Autodesk Inventor part; units mm, degrees
ref_plane "YZ Plane" through (0, 0, 0) normal (1, 0, 0) x (0, 1, 0)
ref_plane "XZ Plane" through (0, 0, 0) normal (0, 1, 0) x (-1, 0, 0)
ref_plane "XY Plane" through (0, 0, 0) normal (0, 0, 1) x (1, 0, 0)
sketch "Sketch1" plane through (0, 0, 0) normal (0, 0, 1) x (1, 0, 0)
  line L0 (-20.935, 3.75) -> (20.935, 3.75)
  line L1 (20.935, 3.75) -> (20.935, -3.75)
  line L2 (20.935, -3.75) -> (-20.935, -3.75)
  line L3 (-20.935, -3.75) -> (-20.935, 3.75)
  line L4 (-20.935, 3.75) -> (20.935, -3.75) construction
  line L5 (20.935, 3.75) -> (-20.935, -3.75) construction
  point P0 (0, 0)
  dimension "d0" = 41.87
  dimension "d1" = 7.5
extrude "Extrusion1" add sketch "Sketch1" along normal mid plane 35.5
sketch "Sketch2" plane through (-20.935, -3.75, 17.75) normal (0, -1, 0) x (1, 0, 0)
  line L0 (0, -35.5) -> (0, 0)
  line L1 (0, -35.5) -> (0, -29.307)
  line L2 (0, -29.307) -> (5, -29.307)
  line L3 (5, -29.307) -> (5, -6.193)
  line L4 (5, -6.193) -> (41.87, -6.193)
  line L5 (41.87, -6.193) -> (41.87, -29.307)
  line L6 (41.87, -29.307) -> (5, -29.307)
  point P0 (20.935, -17.75)
  dimension "d4" = 6.193
  dimension "d5" = 5
  dimension "d6" = 23.114
  dimension "d7" = 36.87
extrude "Extrusion2" cut sketch "Sketch2" against normal blind 1.6
sketch "Sketch3" plane through (-20.935, -2.15, 17.75) normal (0, -1, 0) x (1, 0, 0)
  line L0 (5, -29.307) -> (5, -6.193)
  line L1 (5, -29.307) -> (5, -21.75)
  line L2 (5, -21.75) -> (5, -13.75)
  line L3 (5, -13.75) -> (40, -13.75)
  line L4 (40, -13.75) -> (40, -21.75)
  line L5 (40, -21.75) -> (5, -21.75)
  point P0 (20.935, -17.75)
  dimension "d10" = 7.557
  dimension "d11" = 8
  dimension "d12" = 35
extrude "Extrusion3" cut sketch "Sketch3" against normal blind 1.6
fillet "Fillet1" radius 5 2 edges at (0, 3.75, 17.75) (0, 3.75, -17.75)
fillet "Fillet2" radius 5 5 edges at (20.935, 2.2855, -16.2855) (20.935, -2.5, -17.75) (20.935, 2.2855, 16.2855) (20.935, -2.5, 17.75) (20.935, 3.75, 0)
sketch "Sketch5" plane through (-20.935, -0.55, 17.75) normal (0, -1, 0) x (1, 0, 0)
  line L0 (5, -29.307) -> (5, -21.75)
  line L1 (5, -21.75) -> (5, -20.85)
  line L2 (5, -29.307) -> (5, -6.193)
  line L3 (5, -20.85) -> (7.25, -20.85)
  line L4 (7.25, -20.85) -> (7.25, -14.65)
  line L5 (7.25, -14.65) -> (27.75, -14.65)
  line L6 (27.75, -14.65) -> (27.75, -20.85)
  line L7 (27.75, -20.85) -> (7.25, -20.85)
  point P0 (20.935, -17.75)
  dimension "d22" = 0.9
  dimension "d23" = 2.25
  dimension "d24" = 6.2
  dimension "d25" = 20.5
extrude "Extrusion5" cut sketch "Sketch5" against normal through all
sketch "Sketch6" plane through (-20.935, -3.75, -17.75) normal (0, -1, 0) x (1, 0, 0)
  line L0 (0, 0) -> (0, 35.5)
  line L1 (0, 35.5) -> (-15, 35.5)
  line L2 (-15, 35.5) -> (-15, 0)
  line L3 (-15, 0) -> (0, 0)
  line L4 (0, 0) -> (0, 35.5)
  point P0 (20.935, 17.75)
  dimension "d28" = 15
  dimension "d29" = 35.5
extrude "Extrusion6" add sketch "Sketch6" against normal blind 7.5
fillet "Fillet3" [suppressed]
sketch "Sketch7" plane through (0, 0, 17.75) normal (0, 0, 1) x (1, 0, 0)
  line L0 (-20.9589, -1.4001) -> (-20.9589, -3.75)
  line L1 (15.935, -3.75) -> (-35.935, -3.75)
  line L2 (-35.935, -3.75) -> (-20.9589, -3.75)
  line L3 (-20.9589, -3.75) -> (-20.9589, -14.15)
  line L4 (-20.9589, -14.15) -> (-35.935, -14.15)
  line L5 (-35.935, -14.15) -> (-35.935, -3.75)
  point P0 (0, 0)
  dimension "d33" = 10.4
extrude "Extrusion7" add sketch "Sketch7" against normal blind 35.5
sketch "Sketch8" plane through (0, 0, 17.75) normal (0, 0, 1) x (1, 0, 0)
  line L0 (-35.935, 3.75) -> (-35.935, -14.15)
  line L1 (-35.935, 3.75) -> (-20.935, 3.75)
  arc A0 (-20.935, 3.75) -> (-35.935, -14.15) centre (-14.1441, -17.1757) ccw
  line L2 (-35.935, -14.15) -> (-35.935, 3.75)
  point P0 (0, 0)
  dimension "d36" = 22
extrude "Extrusion8" cut sketch "Sketch8" against normal through all
sketch "Sketch9" plane through (0, 0, 17.75) normal (0, 0, 1) x (1, 0, 0)
  line L0 (-20.9589, -3.75) -> (-20.9589, -14.15)
  line L1 (-20.9589, -3.75) -> (-37.0076, -3.75)
  line L2 (-37.0076, -3.75) -> (-37.0076, -16.8891)
  line L3 (-37.0076, -16.8891) -> (-20.9589, -16.8891)
  line L4 (-20.9589, -16.8891) -> (-20.9589, -3.75)
  point P0 (0, 0)
extrude "Extrusion9" cut sketch "Sketch9" against normal through all
fillet "Fillet4" radius 5 2 edges at (-26.8211, 0.8047, 17.75) (-26.8211, 0.8047, -17.75)
properties part number "Case - Top"
The listing builds one solid part. Answer for the finished solid, in the listing's coordinates (mm). A direction names the side the tool comes from. Coordinates: 2 decimals unless noted, no trailing zeros. Order: outer loops, then holes, each group sorted by start corner. A loop starts at its lowest first (then second) coordinate and runs counter-clockwise, first axis right, second up. Notation, with made-up numbers: M -8.5,36.5 L 33.5,36.5 A13 ccw 33.5,48.5 Z; hole C 31.5,-27.5 d11. An arc over 180 degrees is marked long. Answer as a JSON object with one key per item and string values. Group by question number.
1. Straight lines are drawn through the part: line 1 (Z direction, x = -6, y = -3); line 2 (Z direction, x = 17.5, y = -1.5); line 3 (Y direction, x = 1.5, z = -5). For each, find the intervals that lie inside material, in ascending order.
2. Section A-A on x = 5.5 is taken. Write down the section's boundary in (y, z).
3. Flat-ended cylindrical pins translate along their axes: P1, Ø1.8, axis at y = -1.5, z = 1.5, coming from the -X side; P2, Ø3, axis at y = -0.5, z = -6.5, coming from the -X side; P3, Ø1.3, axis at x = -5.5, y = 1.5, coming from the +Z side. Find the tip coordinate at first contact, or state that the pin passes through.
4. Section D-D on x = 17 is taken. Write down the section's boundary in (y, z).
5. A tool of negligible diameter and unlimited length cuts with its end or side. For faces 4 (the flat face through (3, -3, -11.557)), 5 (the flat face through (-3, 2, -3.1)), 6 (the flat face through (-15.935, -3, 0)), from which of +Z, -Z, +X, -X, +Y, -Y can it reach the whole face along a straight path? Write none if from no direction.
6. Determine the mould class of faces 1 (the cylindrical face through (19.431, -2.518, -16.324)), 2 (the flat face through (-5, -2, 17.75)), 3 (the flat face through (-13.685, 2, 0)) for opening direction X: released by +X, released by -X, zero draft, split by the parting line, or undercut.
Values follow:
{
 "1": {"line 1": "-17.75 to -11.56, 11.56 to 17.75", "line 2": "-17.5 to -4, 4 to 17.5", "line 3": "-2.15 to 3.75"},
 "2": {"outline": "M -3.75,-17.75 L -1.25,-17.75 A5 ccw 3.75,-12.75 L 3.75,-3.1 L -0.55,-3.1 L -0.55,-4 L -2.15,-4 L -2.15,-11.56 L -3.75,-11.56 Z; M -3.75,11.56 L -2.15,11.56 L -2.15,4 L -0.55,4 L -0.55,3.1 L 3.75,3.1 L 3.75,12.75 A5 ccw -1.25,17.75 L -3.75,17.75 Z"},
 "3": {"P1": "x = -30.44", "P2": "x = -30.07", "P3": "z = 17.29"},
 "4": {"outline": "M -3.75,-17.64 L -1.25,-17.64 A4.89 ccw 3.64,-12.75 L 3.64,12.75 A4.89 ccw -1.25,17.64 L -3.75,17.64 L -3.75,11.56 L -2.15,11.56 L -2.15,4 L -0.55,4 L -0.55,-4 L -2.15,-4 L -2.15,-11.56 L -3.75,-11.56 Z"},
 "5": {"face 4": "+X, -Y", "face 5": "+Y, -Y", "face 6": "-Y"},
 "6": {"face 1": "released by +X", "face 2": "zero draft", "face 3": "undercut"}
}
